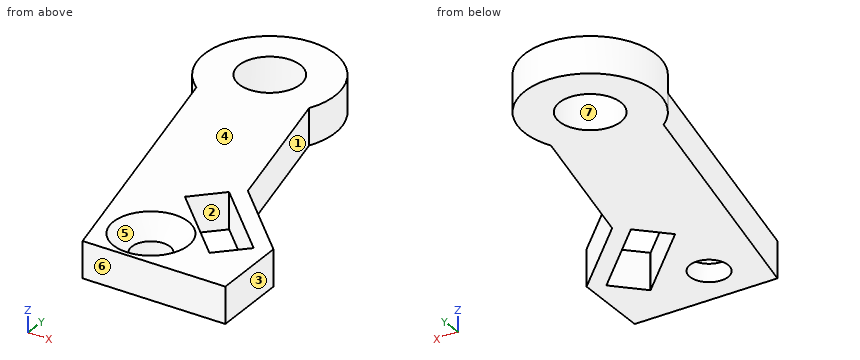
```python
from build123d import *

# Parameters (mm, degrees)
SKETCH1_R           = 1.5
SKETCH1_R_2         = 2.575
BOSS_EXTRUDE1_DEPTH = 3.05


with BuildPart() as part:
    # Sketch1 → Boss-Extrude1 (new body)
    with BuildSketch(Plane.XY):
        with BuildLine():
            Line((-5.003856518, 22.700252006), (0, 0))
            Line((0, 0), (12, 0))
            Line((12, 0), (12, 6.303908615))
            Line((12, 6.303908615), (5.98959236, 12.314316255))
            Line((5.98959236, 12.314316255), (3.296868681, 24.529995477))
            ThreePointArc((3.296868681, 24.529995477), (-2.788944901, 32.395396494), (-5.003856518, 22.700252006))
        make_face()
        with Locations((3.5, 3.5)):
            Circle(SKETCH1_R, mode=Mode.SUBTRACT)
        Polygon((10.727207794, 5.692209589), (8.517499103, 3.482500897), (8.464466094, 3.429467889), (2.701545827, 9.192388155), (4.964287527, 11.455129855), align=None, mode=Mode.SUBTRACT)
        with Locations((-1.604993243, 27.024339012)):
            Circle(SKETCH1_R_2, mode=Mode.SUBTRACT)
    extrude(amount=BOSS_EXTRUDE1_DEPTH)

    # Sketch3 → CSK for M3 Flat Head Machine Screw1 (revolve, cut)
    with BuildSketch(Plane(origin=(3.5, 3.5, 3.05), x_dir=(0, -1, 0), z_dir=(1, 0, 0))):
        Polygon((0, 0), (0, 3.05), (1.6, 3.05), (1.6, 1.55), (3.15, 0), align=None)
    revolve(axis=Axis((3.5, 3.5, 9.4), (0, 0, -1)), mode=Mode.SUBTRACT)


solid = part.part
```
Verification items for the finished model (mm, model axes). Face numbers are marked on the shaded views. A direction names the side the tool comes from. Coordinates: 2 decimals unless noted, no trailing zeros. Write each loop counter-clockwise with the first axis right and the second up, starting at its lowest first coordinate (ties: lowest second). Pieces come first, ordered by that corner, then holes. Notation, with made-up numbers: M 58.25,-24.75 L 98.25,-24.75 A14 cw 98.25,0.25 Z; hole C 85.25,51.5 d2. An arc over 180 degrees is marked long. One line per item, written item: value.
Item 1: Mould release check, pull along Y, two halves, no side actions. Record for the marked faces 4, 5, 6 and 7: pulls with the +Y half, pulls with the -Y half, needs draft (parallel to the pull), parting line crosses it, or undercut.
Check sheet entries:
face 4: needs draft
face 5: undercut
face 6: pulls with the -Y half
face 7: undercut
Item 2: Section check B-B, the plane z = 2.1. State how many separate pieces and enclosed holes the cut face has, plus the area to 3 significant figures.
Check sheet entries:
separate pieces: 1
enclosed holes: 3
area: 266 mm^2
Item 3: Section check A-A, the plane x = 7.25. Record the boundary of the cut face in (y, z).
Check sheet entries:
outline: M 0,0 L 4.64,0 L 4.64,3.05 L 0,3.05 Z; M 9.17,0 L 11.05,0 L 11.05,3.05 L 9.17,3.05 Z
Item 4: Scan lines: line 1 along Y through (x, z) = (3, 0.95); line 2 along Y through (x, z) = (7.5, 2.8); line 3 along X through (y, z) = (3, 0.35). Record each from-to range of solid material in increasing order.
Check sheet entries:
line 1: y = 0 to 1.98, 5.02 to 8.89, 9.49 to 30.03
line 2: y = 0 to 4.39, 8.92 to 10.8
line 3: x = -0.66 to 1.98, 5.02 to 12
Item 5: Access from +Z, -Z, +X, -X, +Y, -Y to the whole of each face (thin tool, end or side, straight path). Record for the marked faces 1, 2 and 3.
Check sheet entries:
face 1: +Z, -Z, +X
face 2: +Z, -Z
face 3: +Z, -Z, +X, +Y, -Y
Item 6: Section check D-D, the plane y = 30.5. Record the boundary of the cut face in (x, z), plus the area to 3 significant figures.
Check sheet entries:
outline: M -5.87,0 L 2.66,0 L 2.66,3.05 L -5.87,3.05 Z
area: 26.0 mm^2
Item 7: Section check C-C, the plane y = 14.5. Record the boundary of the cut face in (x, z), plus the area to 3 significant figures.
Check sheet entries:
outline: M -3.2,0 L 5.51,0 L 5.51,3.05 L -3.2,3.05 Z
area: 26.5 mm^2
